```python
from build123d import *

# Parameters (mm, degrees)
SKETCH_R     = 150
SKETCH_W     = 30
SKETCH_H     = 110
PAD_DEPTH    = 5
FILLET_R     = 3
SKETCH003_R  = 1.25
POCKET_DEPTH = 5.001


with BuildPart() as part:
    # Sketch → Pad (new body)
    with BuildSketch(Plane.XY):
        Circle(SKETCH_R)
        with Locations((-100, 0)):
            Rectangle(SKETCH_W, SKETCH_H, mode=Mode.SUBTRACT)
        with Locations((100, 0)):
            Rectangle(SKETCH_W, SKETCH_H, mode=Mode.SUBTRACT)
    extrude(amount=PAD_DEPTH)

    # Fillet
    fillet_edges = [part.edges().sort_by_distance(p)[0] for p in [
        (-115, -55, 2.5),
        (85, -55, 2.5),
        (115, -55, 2.5),
        (-85, -55, 2.5),
        (115, 55, 2.5),
        (-85, 55, 2.5),
        (-115, 55, 2.5),
        (85, 55, 2.5),
    ]]
    fillet(fillet_edges, radius=FILLET_R)

    # Sketch003 → Pocket (cut, through all)
    with BuildSketch(Plane.XY.offset(5)):
        with Locations((-25, 53.38341)):
            Circle(SKETCH003_R)
        with Locations((25, 53.38341)):
            Circle(SKETCH003_R)
        with Locations((-25, 32.38341)):
            Circle(SKETCH003_R)
        with Locations((25, 32.38341)):
            Circle(SKETCH003_R)
    extrude(amount=-POCKET_DEPTH, mode=Mode.SUBTRACT)


solid = part.part
```
CAD build for the part. Positions are in the model's coordinates, mm. Coordinates: 2 decimals unless noted, no trailing zeros. Write each loop counter-clockwise with the first axis right and the second up, starting at its lowest first coordinate (ties: lowest second). Pieces come first, ordered by that corner, then holes. Notation, with made-up numbers: (-24, 6.25) -> (-18, 6.25) arc R7 cw to (-18, 14.25) -> close; hole circle Ø3 at (48, 83). An arc over 180 degrees is marked (long way). Use CSV: the item, a comma, the result in double quotes. Start each with the question number.
Item 1: Band-saw the part on C-C, the plane z = 1.85. Write the cut outline in (x, y), plus the area to 3 significant figures.
Item 2: Drop flat-ended pins along their axis: P1, Ø2.5, axis at y = 17.5, z = 2.5, coming from the -X side; P2, Ø1.5, axis at x = 94, z = 3.5, coming from the +Y side; P3, Ø1.5, axis at y = -11, z = 2, coming from the -X side. Give the stop position or say it passes through.
Item 3: Band-saw the part on D-D, the plane y = -91.5. Write the cut outline in (x, z), plus the area to 3 significant figures.
Item 4: Band-saw the part on A-A, the plane y = 0. Write the cut outline in (x, z).
Item 5: Band-saw the part on B-B, the plane x = 107. Write the cut outline in (y, z), plus the area to 3 significant figures.
Item 6: Wall check: probe 1 along X at (y, z) = (-32, 4.3); probe 2 along Y at (x, z) = (25, 2.15); probe 3 along X at (y, z) = (-37, 2). Give the ranges that are in metal, low to high.
Response values:
1,outline,"circle Ø300 at (0, 0); hole (-115, -52) arc R3 ccw to (-112, -55) -> (-88, -55) arc R3 ccw to (-85, -52) -> (-85, 52) arc R3 ccw to (-88, 55) -> (-112, 55) arc R3 ccw to (-115, 52) -> close; hole circle Ø2.5 at (-25, 32.38); hole circle Ø2.5 at (-25, 53.38); hole circle Ø2.5 at (25, 32.38); hole circle Ø2.5 at (25, 53.38); hole (85, -52) arc R3 ccw to (88, -55) -> (112, -55) arc R3 ccw to (115, -52) -> (115, 52) arc R3 ccw to (112, 55) -> (88, 55) arc R3 ccw to (85, 52) -> close"
1,area,"64,100 mm2"
2,P1,"stops at x = -149.12"
2,P2,"stops at y = 117.49"
2,P3,"stops at x = -149.65"
3,outline,"(-118.86, 0) -> (118.86, 0) -> (118.86, 5) -> (-118.86, 5) -> close"
3,area,"1,190 mm2"
4,outline,"(-150, 0) -> (-115, 0) -> (-115, 5) -> (-150, 5) -> close; (-85, 0) -> (85, 0) -> (85, 5) -> (-85, 5) -> close; (115, 0) -> (150, 0) -> (150, 5) -> (115, 5) -> close"
5,outline,"(-105.12, 0) -> (-55, 0) -> (-55, 5) -> (-105.12, 5) -> close; (55, 0) -> (105.12, 0) -> (105.12, 5) -> (55, 5) -> close"
5,area,"501 mm2"
6,probe 1,"x = -146.55 to -115, -85 to 85, 115 to 146.55"
6,probe 2,"y = -147.9 to 31.13, 33.63 to 52.13, 54.63 to 147.9"
6,probe 3,"x = -145.37 to -115, -85 to 85, 115 to 145.37"
